from build123d import *

# Parameters (mm, degrees)
SKETCH1_W           = 140
SKETCH1_H           = 160
BOSS_EXTRUDE1_DEPTH = 3
SKETCH2_W           = 120
SKETCH2_H           = 120
SKETCH2_W_2         = 117
SKETCH2_H_2         = 117
BOSS_EXTRUDE2_DEPTH = 70
SKETCH4_W           = 120
SKETCH4_H           = 120
BOSS_EXTRUDE4_DEPTH = 3
SKETCH5_R           = 2.1
SKETCH5_W           = 39.9
SKETCH5_H           = 19.71
CUT_EXTRUDE2_DEPTH  = 3
SKETCH6_W           = 18.298163042
SKETCH6_H           = 17.309993256
CUT_EXTRUDE3_DEPTH  = 3
CUT_EXTRUDE8_DEPTH  = 5
SKETCH15_W          = 259.021634325
SKETCH15_H          = 180.269434884
BOSS_EXTRUDE5_DEPTH = 3
SKETCH18_R          = 1.6
CUT_EXTRUDE9_DEPTH  = 10
SKETCH19_W          = 12
SKETCH19_H          = 4.5
SKETCH19_H_2        = 8.4
SKETCH19_W_2        = 10.084057066
SKETCH19_H_3        = 7.362028533
CUT_EXTRUDE11_DEPTH = 5
SKETCH20_W          = 298.828856564
SKETCH20_H          = 90.290314023
CUT_EXTRUDE12_DEPTH = 233.259150239
SKETCH21_W          = 285.29336792
SKETCH21_H          = 107.84761331
CUT_EXTRUDE13_DEPTH = 210.645587699


with BuildPart() as part:
    # Sketch1 → Boss-Extrude1 (new body)
    with BuildSketch(Plane(origin=(0, 0, 0), x_dir=(1, 0, 0), z_dir=(0, 1, 0))):
        Rectangle(SKETCH1_W, SKETCH1_H)
    extrude(amount=BOSS_EXTRUDE1_DEPTH)

    # Sketch2 → Boss-Extrude2 (add)
    with BuildSketch(Plane(origin=(0, 3, 0), x_dir=(1, 0, 0), z_dir=(0, 1, 0))):
        Rectangle(SKETCH2_W, SKETCH2_H)
        Rectangle(SKETCH2_W_2, SKETCH2_H_2, mode=Mode.SUBTRACT)
    extrude(amount=BOSS_EXTRUDE2_DEPTH)

    # Sketch4 → Boss-Extrude4 (add)
    with BuildSketch(Plane(origin=(0, 73, 0), x_dir=(1, 0, 0), z_dir=(0, 1, 0))):
        Rectangle(SKETCH4_W, SKETCH4_H)
    extrude(amount=BOSS_EXTRUDE4_DEPTH)

    # Sketch5 → Cut-Extrude2 (cut)
    with BuildSketch(Plane(origin=(0, 76, 0), x_dir=(1, 0, 0), z_dir=(0, 1, 0))):
        with Locations(Location((34.39, -4.925, 0), (0, 0, 270))):
            Circle(SKETCH5_R)
        with Locations(Location((34.39, 4.925, 0), (0, 0, 270))):
            Circle(SKETCH5_R)
        with Locations(Location((-15.03, -4.925, 0), (0, 0, 270))):
            Circle(SKETCH5_R)
        with Locations(Location((-15.03, 4.925, 0), (0, 0, 270))):
            Circle(SKETCH5_R)
        with Locations((9.68, 0)):
            Rectangle(SKETCH5_W, SKETCH5_H)
    extrude(amount=-CUT_EXTRUDE2_DEPTH, mode=Mode.SUBTRACT)

    # Sketch6 → Cut-Extrude3 (cut)
    with BuildSketch(Plane(origin=(0, 76, 0), x_dir=(1, 0, 0), z_dir=(0, 1, 0))):
        Rectangle(SKETCH6_W, SKETCH6_H)
    extrude(amount=-CUT_EXTRUDE3_DEPTH, mode=Mode.SUBTRACT)

    # Sketch13 → Cut-Extrude8 (cut)
    with BuildSketch(Plane(origin=(0, 76, 0), x_dir=(1, 0, 0), z_dir=(0, 1, 0))):
        with BuildLine():
            ThreePointArc((-3.792582359, 49.728765052), (-53.491503795, -1.722579942), (-0.349490011, -49.609426409))
            ThreePointArc((-0.349490011, -49.609426409), (5.82592347, -42.51288634), (-1.270616599, -36.337472859))
            ThreePointArc((-1.270616599, -36.337472859), (-40.195607742, -1.261740085), (-3.792582359, 36.42488497))
            ThreePointArc((-3.792582359, 36.42488497), (2.859357682, 43.076825011), (-3.792582359, 49.728765052))
        make_face()
    extrude(amount=-CUT_EXTRUDE8_DEPTH, mode=Mode.SUBTRACT)

    # Sketch15 → Boss-Extrude5 (add)
    with BuildSketch(Plane(origin=(0, 3, 0), x_dir=(1, 0, 0), z_dir=(0, 1, 0))):
        with Locations((-39.510817163, -10.134717442)):
            Rectangle(SKETCH15_W, SKETCH15_H)
    extrude(amount=-BOSS_EXTRUDE5_DEPTH)

    # Sketch18 → Cut-Extrude9 (cut)
    with BuildSketch(Plane(origin=(0, 3, 0), x_dir=(1, 0, 0), z_dir=(0, 1, 0))):
        with Locations(Location((-55.452, -27.227420358, 0), (0, 0, 270))):
            Circle(SKETCH18_R)
        with Locations(Location((-55.452, 32.208579642, 0), (0, 0, 270))):
            Circle(SKETCH18_R)
        with Locations(Location((4.746, 32.208579642, 0), (0, 0, 270))):
            Circle(SKETCH18_R)
        with Locations(Location((4.746, -27.227420358, 0), (0, 0, 270))):
            Circle(SKETCH18_R)
    extrude(amount=-CUT_EXTRUDE9_DEPTH, mode=Mode.SUBTRACT)

    # Sketch19 → Cut-Extrude11 (cut)
    with BuildSketch(Plane.ZY.offset(60)):
        with Locations((12.367420358, 33)):
            Rectangle(SKETCH19_W, SKETCH19_H)
        with Locations((-11.259414931, 37.2)):
            Rectangle(SKETCH19_W, SKETCH19_H_2)
        with Locations((-28.606781654, 36.742945388)):
            Rectangle(SKETCH19_W_2, SKETCH19_H_3)
    extrude(amount=-CUT_EXTRUDE11_DEPTH, mode=Mode.SUBTRACT)

    # Sketch20 → Cut-Extrude12 (cut, through all)
    with BuildSketch(Plane.XY.offset(60)):
        with Locations((-35.656907555, 27.854842988)):
            Rectangle(SKETCH20_W, SKETCH20_H)
    extrude(amount=-CUT_EXTRUDE12_DEPTH, mode=Mode.SUBTRACT)


with BuildPart() as cut_extrude12_piece_1:
    # of the separate pieces the step leaves, piece 1, a body of its own (cut_extrude12_pieces)
    add(part.part.solids().sort_by_distance((60, 76, 60))[0])


with BuildPart() as cut_extrude12_piece_2:
    # of the separate pieces the step leaves, piece 2, a body of its own (cut_extrude12_pieces)
    add(part.part.solids().sort_by_distance((90, 0, 60))[0])

    # Sketch21 → Cut-Extrude13 (cut, through all)
    with BuildSketch(Plane(origin=(0, 3, 0), x_dir=(1, 0, 0), z_dir=(0, 1, 0))):
        with Locations((-30.056705319, -107.088557651)):
            Rectangle(SKETCH21_W, SKETCH21_H)
    extrude(amount=-CUT_EXTRUDE13_DEPTH, mode=Mode.SUBTRACT)


solid = cut_extrude12_piece_1.part
Can you work these out from the model? Positions are in its coordinate system, mm. A direction names the side the tool comes from. Coordinates: 2 decimals unless noted, no trailing zeros. Write each loop counter-clockwise with the first axis right and the second up, starting at its lowest first coordinate (ties: lowest second). Pieces come first, ordered by that corner, then holes. Notation, with made-up numbers: (-32.75, -17.5) -> (-1.75, -17.5) arc R21 ccw to (-1.75, 7.5) -> close; hole circle Ø6 at (36.25, -25.5). An arc over 180 degrees is marked (long way). Write item = value, one per line.
(1) Imagine slicing it at A-A (z = 0). Please give me the cut outline in (x, y).
Verdict:
outline = (-60, 73) -> (-53.52, 73) -> (-53.52, 76) -> (-60, 76) -> close; (-40.22, 73) -> (-10.27, 73) -> (-10.27, 76) -> (-40.22, 76) -> close; (29.63, 73) -> (60, 73) -> (60, 76) -> (29.63, 76) -> close
(2) Imagine slicing it at B-B (x = 10). Please give me the cut outline in (y, z) (3 decimals).
Verdict:
outline = (73, -60) -> (76, -60) -> (76, -9.855) -> (73, -9.855) -> close; (73, 9.855) -> (76, 9.855) -> (76, 60) -> (73, 60) -> close
(3) Imagine slicing it at C-C (x = 34.39). Please give me the cut outline in (y, z) (3 decimals), and give its area (3 significant figures).
Verdict:
outline = (73, -60) -> (76, -60) -> (76, -7.025) -> (73, -7.025) -> close; (73, -2.825) -> (76, -2.825) -> (76, 2.825) -> (73, 2.825) -> close; (73, 7.025) -> (76, 7.025) -> (76, 60) -> (73, 60) -> close
area = 335 mm^2
(4) Thinking about a two-plate mould opening in Z: for faces 3 (the face through (-60, 74, 1)), 4 (the face through (9, 75, 9.855)), 5 (the face through (-1, 74, 60)), 6 (the face through (-1, 74, -60)), which applies, +Z half, -Z half, draft (parallel to the pull), parting line (faces both ways), or undercut?
Verdict:
face_3 = draft
face_4 = undercut
face_5 = +Z half
face_6 = -Z half
(5) On a 3-axis mill with a long thin cutter (end or side, diameter ignored), from which of +Z, -Z, +X, -X, +Y, -Y can I reach the whole of each face in a straight line? I mean faces 1 (the face through (2.858, 74.521, -42.931)), 2 (the face through (60, 74, 1)). Say none if no direction works.
Verdict:
face_1 = +Y, -Y
face_2 = +Z, -Z, +X, +Y, -Y
(6) If I drill on probe 1 along Z at (x, y) = (13, 74.8) (3 decimals); probe 2 along Z at (x, y) = (-17.5, 74.15); probe 3 along X at (y, z) = (73.3, 5), over which ranges is the centre line in solid material (lowest first)?
Verdict:
probe_1 = -60 to -9.855, 9.855 to 60
probe_2 = -60 to -47.8, -33.75 to 33.75, 47.8 to 60
probe_3 = -60 to -53.27, -39.87 to -17.13, -12.93 to -10.27, 29.63 to 32.29, 36.49 to 60
(7) Imagine slicing it at D-D (z = 21). Please give me the cut outline in (x, y).
Verdict:
outline = (-60, 73) -> (-48.87, 73) -> (-48.87, 76) -> (-60, 76) -> close; (-33.55, 73) -> (60, 73) -> (60, 76) -> (-33.55, 76) -> close
